from build123d import *

# Parameters (mm, degrees)
ESBO_O1_W                = 50
ESBO_O1_H                = 112
RESSALTO_EXTRUS_O1_DEPTH = 6
ESBO_O2_W                = 20
ESBO_O2_H                = 6
CORTE_EXTRUS_O1_DEPTH    = 6
ESBO_O5_R                = 1.75
CORTE_EXTRUS_O3_DEPTH    = 6


with BuildPart() as part:
    # Esboço1 → Ressalto-extrusão1 (new body)
    with BuildSketch(Plane(origin=(0, 0, 0), x_dir=(1, 0, 0), z_dir=(0, 1, 0))):
        with Locations((-22.136094675, 56)):
            Rectangle(ESBO_O1_W, ESBO_O1_H)
    extrude(amount=RESSALTO_EXTRUS_O1_DEPTH)

    # Esboço2 → Corte-extrusão1 (cut)
    with BuildSketch(Plane.XY):
        with Locations((-37.136094675, 3)):
            Rectangle(ESBO_O2_W, ESBO_O2_H)
        with Locations((-7.136094675, 3)):
            Rectangle(ESBO_O2_W, ESBO_O2_H)
    extrude(amount=-CORTE_EXTRUS_O1_DEPTH, mode=Mode.SUBTRACT)

    # Esboço5 → Corte-extrusão3 (cut)
    with BuildSketch(Plane(origin=(0, 6, 0), x_dir=(1, 0, 0), z_dir=(0, 1, 0))):
        with Locations(Location((-42.136094675, 104.5, 0), (0, 0, 270))):
            Circle(ESBO_O5_R)
        with Locations(Location((-42.136094675, 89.5, 0), (0, 0, 270))):
            Circle(ESBO_O5_R)
        with Locations(Location((-42.136094675, 74.5, 0), (0, 0, 270))):
            Circle(ESBO_O5_R)
        with Locations(Location((-42.136094675, 59.5, 0), (0, 0, 270))):
            Circle(ESBO_O5_R)
        with Locations(Location((-42.136094675, 44.5, 0), (0, 0, 270))):
            Circle(ESBO_O5_R)
        with Locations(Location((-42.136094675, 13.5, 0), (0, 0, 270))):
            Circle(ESBO_O5_R)
        with Locations(Location((-42.136094675, 29.5, 0), (0, 0, 270))):
            Circle(ESBO_O5_R)
        with Locations(Location((-2.136094675, 104.491725396, 0), (0, 0, 270))):
            Circle(ESBO_O5_R)
        with Locations(Location((-2.136094675, 89.491725396, 0), (0, 0, 270))):
            Circle(ESBO_O5_R)
        with Locations(Location((-2.136094675, 74.491725396, 0), (0, 0, 270))):
            Circle(ESBO_O5_R)
        with Locations(Location((-2.136094675, 59.491725396, 0), (0, 0, 270))):
            Circle(ESBO_O5_R)
        with Locations(Location((-2.136094675, 44.491725396, 0), (0, 0, 270))):
            Circle(ESBO_O5_R)
        with Locations(Location((-2.136094675, 13.491725396, 0), (0, 0, 270))):
            Circle(ESBO_O5_R)
        with Locations(Location((-2.136094675, 29.491725396, 0), (0, 0, 270))):
            Circle(ESBO_O5_R)
    extrude(amount=-CORTE_EXTRUS_O3_DEPTH, mode=Mode.SUBTRACT)


solid = part.part
Geometry check sheet. Reference: the model listing, model coordinates, mm. A direction names the side the tool comes from. Round coordinates to 2 decimals unless told otherwise and drop trailing zeros. Write each loop counter-clockwise with the first axis right and the second up, starting at its lowest first coordinate (ties: lowest second). Pieces come first, ordered by that corner, then holes.
Item 1: Go/stop test with a flat-tipped pin: pin 1 Ø4.5 at (x, z) = (-42.14, -44.5) entering from -Y. Record where the tip stops, or that it passes through.
Determined:
pin 1: stops at y = 0
Item 2: Mould release check, pull along Z, two halves, no side actions. Record for faces 3 (the face through (-7, 3, -6)), 4 (the face through (-17.136, 3, -3)), 5 (the face through (-2.06, 3.04, -106.24)): +Z half, -Z half, draft (parallel to the pull), parting line (faces both ways), or undercut.
Determined:
face 3: +Z half
face 4: draft
face 5: undercut
Item 3: Access from +Z, -Z, +X, -X, +Y, -Y to the whole of each face (thin tool, end or side, straight path). Record for faces 1 (the face through (-37, 3, -6)), 2 (the face through (-41.61, 3.04, -72.83)).
Determined:
face 1: +Z, -X, +Y, -Y
face 2: +Y, -Y
Item 4: Section check A-A (y = 3.55). Give the number of separate pieces and of enclosed holes in the cut face, plus the area to 3 significant figures.
Determined:
separate pieces: 1
enclosed holes: 14
area: 5,230 mm2
Item 5: Section check B-B (z = -29.5). Record the boundary of the cut face in (x, y), plus the area to 3 significant figures.
Determined:
outline: (-47.14, 0) - (-43.89, 0) - (-43.89, 6) - (-47.14, 6) - close; (-40.39, 0) - (-3.89, 0) - (-3.89, 6) - (-40.39, 6) - close; (-0.39, 0) - (2.86, 0) - (2.86, 6) - (-0.39, 6) - close
area: 258 mm2
Item 6: Section check C-C (x = -16). Record the boundary of the cut face in (y, z), plus the area to 3 significant figures.
Determined:
outline: (0, -112) - (6, -112) - (6, -6) - (0, -6) - close
area: 636 mm2
Item 7: Material ranges on line 1 along X through (y, z) = (1.3, -89.5); line 2 along X through (y, z) = (2.95, -103); line 3 along Z through (x, y) = (-29.5, 2.15), recorded low to high.
Determined:
line 1: x = -47.14 to -43.89, -40.39 to -3.89, -0.39 to 2.86
line 2: x = -47.14 to -43.04, -41.23 to -3.05, -1.22 to 2.86
line 3: z = -112 to -6
